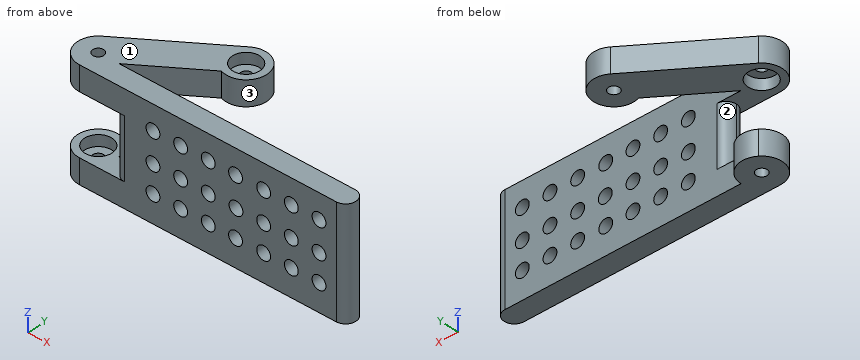
```python
from build123d import *

# Parameters (mm, degrees)
SKETCH1_R           = 2
BOSS_EXTRUDE1_DEPTH = 40
SKETCH2_W           = 20
SKETCH2_H           = 22
CUT_EXTRUDE1_DEPTH  = 38.943057454
SKETCH3_R           = 2
CUT_EXTRUDE2_DEPTH  = 31
FILLET1_R           = 3.7
SKETCH4_R           = 2.5
CUT_EXTRUDE3_DEPTH  = 30
SKETCH5_R           = 5
CUT_EXTRUDE4_DEPTH  = 4
SKETCH11_R          = 5
CUT_EXTRUDE6_DEPTH  = 4
SKETCH12_R          = 5
CUT_EXTRUDE7_DEPTH  = 4


with BuildPart() as part:
    # Sketch1 → Boss-Extrude1 (new body)
    with BuildSketch(Plane.XY):
        with BuildLine():
            Line((28.464258499, 29.086697786), (-4.301823273, 6.143640332))
            ThreePointArc((-4.301823273, 6.143640332), (-7.152877131, -2.255293496), (0, -7.5))
            Line((0, -7.5), (92.766081772, -7.5))
            ThreePointArc((92.766081772, -7.5), (96.516081772, -3.75), (92.766081772, 0))
            Line((92.766081772, 0), (7.5, 0))
            Line((7.5, 0), (30.200930697, 15.895362798))
            ThreePointArc((30.200930697, 15.895362798), (40.201918232, 23.922003896), (28.464258499, 29.086697786))
        make_face()
        with Locations((32.766081772, 22.943057454)):
            Circle(SKETCH1_R, mode=Mode.SUBTRACT)
        Circle(SKETCH1_R, mode=Mode.SUBTRACT)
    extrude(amount=BOSS_EXTRUDE1_DEPTH)

    # Sketch2 → Cut-Extrude1 (cut, through all)
    with BuildSketch(Plane.XZ.offset(7.5)):
        with Locations((2.5, 20)):
            Rectangle(SKETCH2_W, SKETCH2_H)
    extrude(amount=-CUT_EXTRUDE1_DEPTH, mode=Mode.SUBTRACT)

    # Sketch3 → Cut-Extrude2 (cut)
    with BuildSketch(Plane(origin=(0, 0, 0), x_dir=(-1, 0, 0), z_dir=(0, 0, -1))):
        with BuildLine():
            Line((-30.200930697, 15.895362798), (-7.5, 0))
            ThreePointArc((-7.5, 0), (-3.463114599, 6.652581249), (4.301823273, 6.143640332))
            Line((4.301823273, 6.143640332), (-28.464258499, 29.086697786))
            ThreePointArc((-28.464258499, 29.086697786), (-40.201918232, 23.922003896), (-30.200930697, 15.895362798))
        make_face()
        with Locations((-32.766081772, 22.943057454)):
            Circle(SKETCH3_R, mode=Mode.SUBTRACT)
    extrude(amount=-CUT_EXTRUDE2_DEPTH, mode=Mode.SUBTRACT)

    # Fillet1
    fillet1_edges = [part.edges().sort_by_distance(p)[0] for p in [
        (12.5, 0, 20),
        (12.5, -7.5, 20),
    ]]
    fillet(fillet1_edges, radius=FILLET1_R)

    # Sketch4 → Cut-Extrude3 (cut)
    with BuildSketch(Plane(origin=(0, 0, 0), x_dir=(1, 0, 0), z_dir=(0, 1, 0))):
        with Locations((86.516081772, -10)):
            Circle(SKETCH4_R)
        with Locations((86.516081772, -20)):
            Circle(SKETCH4_R)
        with Locations((86.516081772, -31)):
            Circle(SKETCH4_R)
        with Locations((76.516081772, -31)):
            Circle(SKETCH4_R)
        with Locations((76.516081772, -20)):
            Circle(SKETCH4_R)
        with Locations((76.516081772, -10)):
            Circle(SKETCH4_R)
        with Locations((66.516081772, -10)):
            Circle(SKETCH4_R)
        with Locations((66.516081772, -20)):
            Circle(SKETCH4_R)
        with Locations((66.516081772, -31)):
            Circle(SKETCH4_R)
        with Locations((56.358040886, -31)):
            Circle(SKETCH4_R)
        with Locations((56.516081772, -20)):
            Circle(SKETCH4_R)
        with Locations((56.358040886, -10)):
            Circle(SKETCH4_R)
        with Locations((46.516081772, -10)):
            Circle(SKETCH4_R)
        with Locations((46.516081772, -20)):
            Circle(SKETCH4_R)
        with Locations((46.516081772, -31)):
            Circle(SKETCH4_R)
        with Locations((36.516081772, -31)):
            Circle(SKETCH4_R)
        with Locations((36.516081772, -20)):
            Circle(SKETCH4_R)
        with Locations((36.516081772, -10)):
            Circle(SKETCH4_R)
        with Locations((26.516081772, -10)):
            Circle(SKETCH4_R)
        with Locations((26.516081772, -20)):
            Circle(SKETCH4_R)
        with Locations((26.516081772, -31)):
            Circle(SKETCH4_R)
    extrude(amount=-CUT_EXTRUDE3_DEPTH, mode=Mode.SUBTRACT)

    # Sketch5 → Cut-Extrude4 (cut)
    with BuildSketch(Plane.XY.offset(9)):
        Circle(SKETCH5_R)
    extrude(amount=-CUT_EXTRUDE4_DEPTH, mode=Mode.SUBTRACT)

    # Sketch11 → Cut-Extrude6 (cut)
    with BuildSketch(Plane(origin=(0, 0, 31), x_dir=(-1, 0, 0), z_dir=(0, 0, -1))):
        Circle(SKETCH11_R)
    extrude(amount=-CUT_EXTRUDE6_DEPTH, mode=Mode.SUBTRACT)

    # Sketch12 → Cut-Extrude7 (cut)
    with BuildSketch(Plane.XY.offset(40)):
        with Locations((32.766081772, 22.943057454)):
            Circle(SKETCH12_R)
    extrude(amount=-CUT_EXTRUDE7_DEPTH, mode=Mode.SUBTRACT)


solid = part.part
```
Check sheet for the modelled part. Datum: model origin and axes. Units: mm. Face numbers are marked on the shaded views. Give positions to 0.01 mm unless a question says otherwise; leave off trailing zeros. Order: outer loops, then holes, each group sorted by start corner. A loop starts at its lowest first (then second) coordinate and runs counter-clockwise, first axis right, second up. Notation, with made-up numbers: M 83.5,80 L 103.5,80 A26 cw 103.5,96 Z; hole C 0,-38.5 d7. An arc over 180 degrees is marked long. Answer in a Markdown table with one row per item.
1) Cross-section at B-B, the plane x = 85. Enter the section's corners in (y, z).
Filled sheet:
| item | result |
|---|---|
| outline | M -7.5,0 L 0,0 L 0,8.01 L -7.5,8.01 Z; M -7.5,11.99 L 0,11.99 L 0,18.01 L -7.5,18.01 Z; M -7.5,21.99 L 0,21.99 L 0,29.01 L -7.5,29.01 Z; M -7.5,32.99 L 0,32.99 L 0,40 L -7.5,40 Z |
2) Thickness scan on L1, parallel to Z at x = 66, y = -1; L2, parallel to Z at x = 14, y = 6; L3, parallel to Y at x = 12, z = 3. Record the ranges inside material, lowest first. Write a range as [from, to].
Filled sheet:
| item | result |
|---|---|
| L1 | z = [0, 7.55], [12.45, 17.55], [22.45, 28.55], [33.45, 40] |
| L2 | z = [31, 40] |
| L3 | y = [-7.5, 0] |
3) Release check for a two-part mould opening along Z. For the marked faces 1, 2 and 3 record: +Z half, -Z half, draft (parallel to the pull), parting line (faces both ways), or undercut.
Filled sheet:
| item | result |
|---|---|
| face 1 | +Z half |
| face 2 | undercut |
| face 3 | draft |
4) Gauge pin test, flat ends, axial feed: P1, Ø4, axis at x = 26.52, z = 10, coming from the -Y side; P2, Ø6.5, axis at x = 36.52, z = 10, coming from the +Y side; P3, Ø6, axis at y = 24.5, z = 32.5, coming from the +X side; P4, Ø19, axis at x = 11.5, y = 13.5, coming from the -Z side. Record the tip position at first contact, or that the pin passes through.
Filled sheet:
| item | result |
|---|---|
| P1 | passes through |
| P2 | stops at y = 0 |
| P3 | stops at x = 40.27 |
| P4 | stops at z = 31 |
5) Cross-section at C-C, the plane z = 26. Enter the section's corners in (x, y).
Filled sheet:
| item | result |
|---|---|
| outline | M 12.5,-3.8 A3.7 ccw 16.2,-7.5 L 92.77,-7.5 A3.75 ccw 92.77,0 L 16.2,0 A3.7 ccw 12.5,-3.7 Z |
6) Cross-section at A-A, the plane z = 20. Count the separate pieces of the cut face and the enclosed holes in it, plus the area to 3 significant figures.
Filled sheet:
| item | result |
|---|---|
| separate pieces | 8 |
| enclosed holes | 0 |
| area | 356 mm2 |
